```python
from build123d import *

# Parameters (mm, degrees)
SKETCH1_W           = 40
SKETCH1_H           = 16.8
SKETCH1_R           = 1.5
BOSS_EXTRUDE1_DEPTH = 2
FILLET1_R           = 10


with BuildPart() as part:
    # Sketch1 → Boss-Extrude1 (new body)
    with BuildSketch(Plane(origin=(0, 0, 0), x_dir=(1, 0, 0), z_dir=(0, 1, 0))):
        Rectangle(SKETCH1_W, SKETCH1_H)
        with Locations(Location((-11, 0, 0), (0, 0, 270))):
            Circle(SKETCH1_R, mode=Mode.SUBTRACT)
        with Locations(Location((1, 0, 0), (0, 0, 270))):
            Circle(SKETCH1_R, mode=Mode.SUBTRACT)
        with Locations(Location((13, 0, 0), (0, 0, 270))):
            Circle(SKETCH1_R, mode=Mode.SUBTRACT)
    extrude(amount=BOSS_EXTRUDE1_DEPTH)

    # Fillet1
    # the kernel refuses this fillet: 10 mm, written as the material it takes off along each edge
    with BuildSketch(Plane(origin=(20, -25, -8.4), x_dir=(0, 0, 1), z_dir=(0, 1, 0)), Plane(origin=(20, -25, 8.4), x_dir=(-1, 0, 0), z_dir=(0, 1, 0))) as fillet1_piece_1:
        with BuildLine():
            CenterArc((FILLET1_R, -FILLET1_R), FILLET1_R, 90, 90)
            Line((0, -FILLET1_R), (0, 0))
            Line((0, 0), (FILLET1_R, 0))
        make_face()
    extrude(amount=52, mode=Mode.SUBTRACT)


solid = part.part
```
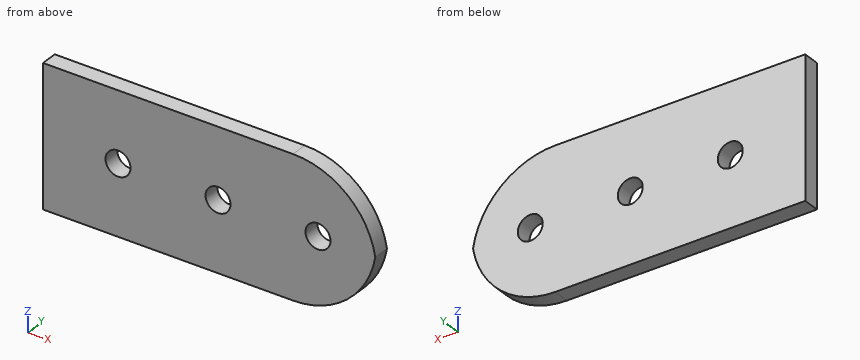
Geometry check sheet. Reference: the model listing, model coordinates, mm. Coordinates: 2 decimals unless noted, no trailing zeros. Order: outer loops, then holes, each group sorted by start corner. A loop starts at its lowest first (then second) coordinate and runs counter-clockwise, first axis right, second up. Notation, with made-up numbers: M -14,18.5 L 4,18.5 A23 ccw 4,27.5 Z; hole C 12,63 d7. An arc over 180 degrees is marked long. Answer as a JSON object with one key per item and string values.
Q1. Scan lines: line 1 (Z direction, x = -11.5, y = 1.65); line 2 (Z direction, x = 2, y = 1.4); line 3 (X direction, y = 1.45, z = -6.5). Record each from-to range of solid material in increasing order.
Results are:
{"line 1": "z = -8.4 to -1.41, 1.41 to 8.4", "line 2": "z = -8.4 to -1.12, 1.12 to 8.4", "line 3": "x = -20 to 15.86"}
Q2. Cross-section at A-A on x = -11. Record the cut outline in (y, z).
Results are:
{"outline": "M 0,-8.4 L 2,-8.4 L 2,-1.5 L 0,-1.5 Z; M 0,1.5 L 2,1.5 L 2,8.4 L 0,8.4 Z"}
Q3. Cross-section at C-C on x = 0. Record the cut outline in (y, z).
Results are:
{"outline": "M 0,-8.4 L 2,-8.4 L 2,-1.12 L 0,-1.12 Z; M 0,1.12 L 2,1.12 L 2,8.4 L 0,8.4 Z"}
Q4. Cross-section at D-D on z = 7.75. Record the cut outline in (x, y).
Results are:
{"outline": "M -20,0 L 13.55,0 L 13.55,2 L -20,2 Z"}
Q5. Cross-section at B-B on y = 1.7. Record the cut outline in (x, z).
Results are:
{"outline": "M -20,-8.4 L 10,-8.4 A10 ccw 19.87,0 A10 ccw 10,8.4 L -20,8.4 Z; hole C -11,0 d3; hole C 1,0 d3; hole C 13,0 d3"}
